For this review, use the dimensioned drawing (mm, ordinates from the lowest corner) and the shaded views. A direction names the side the tool comes from. Give positions to 0.01 mm unless a question says otherwise; leave off trailing zeros. Order: outer loops, then holes, each group sorted by start corner. A loop starts at its lowest first (then second) coordinate and runs counter-clockwise, first axis right, second up. Notation, with made-up numbers: (45, 64) -> (76, 64) arc R15 cw to (76, 79) -> close; hole circle Ø9 at (44, 4.25). An arc over 180 degrees is marked (long way). Return JSON: item names as keys, results as strings.
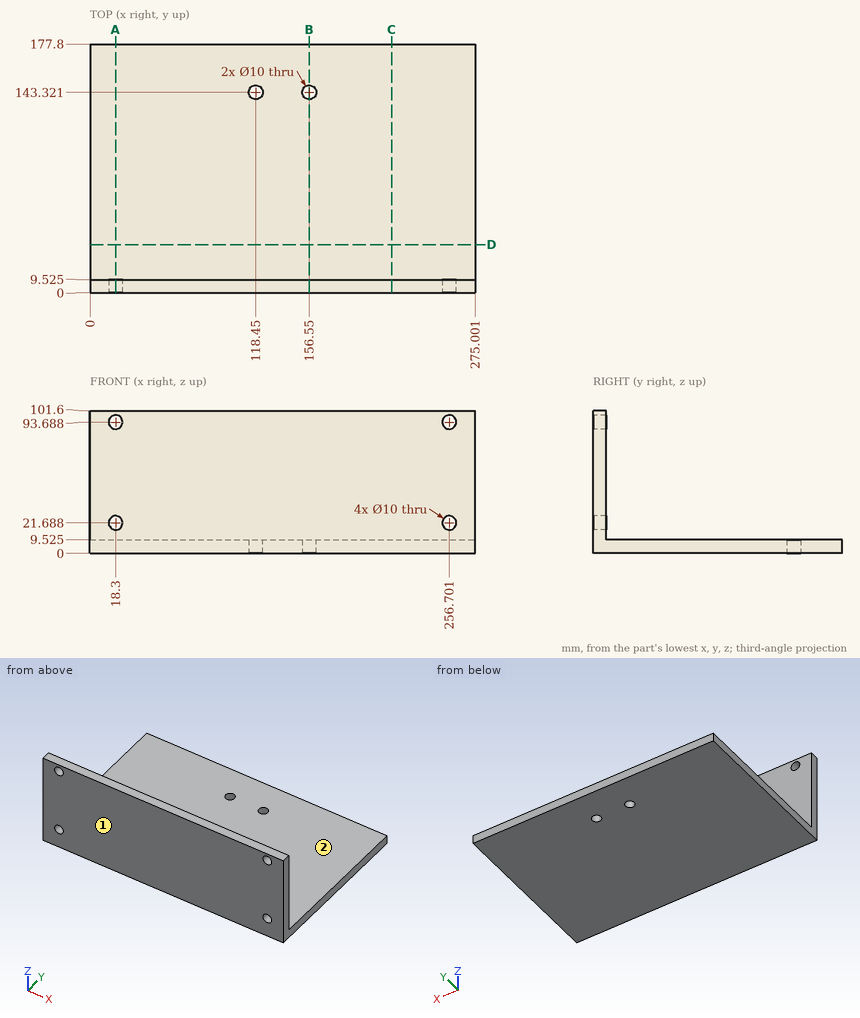
Item 1: Add section B-B (x = 156.5). Give the boundary of the cut face in (y, z) (1 decimal).
Result set:
{"outline": "(0, 0) -> (138.3, 0) -> (138.3, 9.5) -> (9.5, 9.5) -> (9.5, 101.6) -> (0, 101.6) -> close; (148.3, 0) -> (177.8, 0) -> (177.8, 9.5) -> (148.3, 9.5) -> close"}
Item 2: Machinability: for the marked faces 1 and 2, which of the approach directions +Z, -Z, +X, -X, +Y, -Y give a long, thin tool a straight path to every point of the face, cutting with its end or side? Answer none if there is none.
Result set:
{"face 1": "+Z, -Z, +X, -X, -Y", "face 2": "+Z, +X, -X, +Y"}
Item 3: Add section A-A (x = 18.3). Give the boundary of the cut face in (y, z) (1 decimal).
Result set:
{"outline": "(0, 0) -> (177.8, 0) -> (177.8, 9.5) -> (9.5, 9.5) -> (9.5, 16.7) -> (0, 16.7) -> close; (0, 26.7) -> (9.5, 26.7) -> (9.5, 88.7) -> (0, 88.7) -> close; (0, 98.7) -> (9.5, 98.7) -> (9.5, 101.6) -> (0, 101.6) -> close"}
Item 4: Add section D-D (y = 34.5). Give the boundary of the cut face in (x, z) (1 decimal).
Result set:
{"outline": "(0, 0) -> (275, 0) -> (275, 9.5) -> (0, 9.5) -> close"}
Item 5: For pin 1 (16 mm diameter, centred on x = 256.7, z = 93.69, fed in from +Y) (1 decimal); pin 2 (3 mm diameter, centred on x = 172.5, y = 153.5, fed in from +Z) (1 decimal), all flat-tipped, find the tip position at first contact; note any pin that passes through.
Result set:
{"pin 1": "stops at y = 9.5", "pin 2": "stops at z = 9.5"}
Item 6: Add section C-C (x = 215.5). Give the boundary of the cut face in (y, z) (1 decimal), plus the area to 3 significant figures.
Result set:
{"outline": "(0, 0) -> (177.8, 0) -> (177.8, 9.5) -> (9.5, 9.5) -> (9.5, 101.6) -> (0, 101.6) -> close", "area": "2,570 mm^2"}
Item 7: Wall thickness on L1, parallel to Z at x = 18.3, y = 4; L2, parallel to Y at x = 233, z = 62.5 (1 decimal): over which ranges is each line inside the solid? List them lowest first. Write a range as [from, to].
Result set:
{"L1": "z = [0, 16.69], [26.69, 88.69], [98.69, 101.6]", "L2": "y = [0, 9.5]"}
